Answer from the drawing. Dimensions are ordinates in mm from the lowest x, y and z of the part. A direction names the side the tool comes from. Give positions to 0.01 mm unless a question says otherwise; leave off trailing zeros. Loops run counter-clockwise (first coordinate to the right, second up) from the corner with the lowest first, then second, coordinate; pieces in that order, holes last.
Item 1: Section C-C, the plane z = 2 is taken. Give the vertices of the cut face in (x, y).
Item 2: Section D-D, the plane x = 58.5 is taken. Give the vertices of the cut face in (y, z), and give its area (3 significant figures).
Item 3: Section A-A, the plane y = 11.5 is taken. Give the vertices of the cut face in (x, z), and give its area (3 significant figures).
Item 4: Section B-B, the plane z = 9 is taken. Give the vertices of the cut face in (x, y).
Item 5: Consider line 1 along X through (y, z) = (28.5, 2.5); line 2 along Y through (x, z) = (72, 2.5); line 3 along X through (y, z) = (23.5, 7). Determine where each line is inside the solid, lowest interval first.
Item 6: The mould has two halves that part along X. Classify the marked faces 1, 2, 3 and 4: pulls with the +X half, pulls with the -X half, needs draft (parallel to the pull), parting line crosses it, or undercut.
Item 7: Each of these flat-tipped pins is pushed along its axis until it touches: pin 1 Ø4 at (x, y) = (72, 6.5) entering from +Z; pin 2 Ø6 at (y, z) = (25, 4.5) entering from +X; pin 3 Ø3 at (x, z) = (3.5, 5) entering from +Y (3 decimals); pin 4 Ø3 at (y, z) = (16.5, 5) entering from +X. Where does it stop, or does it pass through?
Item 8: A tool of negligible diameter and unlimited length cuts with its end or side. For the marked faces 5, 6, 7, 8 and 9, from which of +Z, -Z, +X, -X, +Y, -Y can it reach the whole face along a straight path? Write none if from no direction.
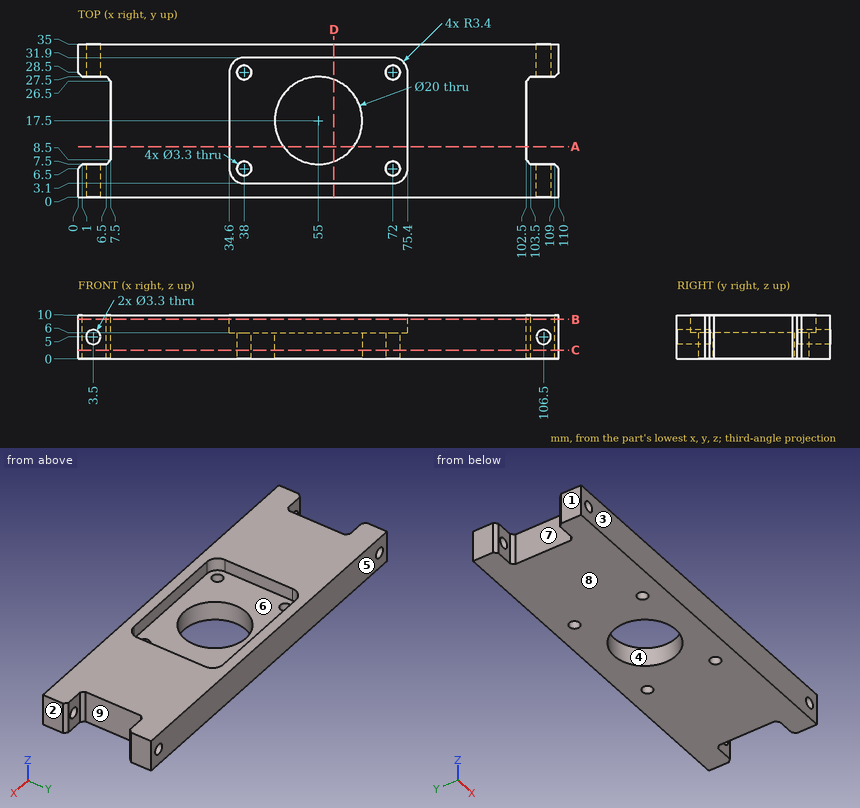
Worked answers:
1. outline: (0, 0) - (110, 0) - (110, 6.5) - (109, 7.5) - (103.5, 7.5) - (102.5, 8.5) - (102.5, 26.5) - (103.5, 27.5) - (109, 27.5) - (110, 28.5) - (110, 35) - (0, 35) - (0, 28.5) - (1, 27.5) - (6.5, 27.5) - (7.5, 26.5) - (7.5, 8.5) - (6.5, 7.5) - (1, 7.5) - (0, 6.5) - close; hole circle Ø3.3 at (38, 6.5); hole circle Ø3.3 at (38, 28.5); hole circle Ø20 at (55, 17.5); hole circle Ø3.3 at (72, 6.5); hole circle Ø3.3 at (72, 28.5)
2. outline: (0, 0) - (8.13, 0) - (8.13, 6) - (3.1, 6) - (3.1, 10) - (0, 10) - close; (26.87, 0) - (35, 0) - (35, 10) - (31.9, 10) - (31.9, 6) - (26.87, 6) - close
2. area: 122 mm2
3. outline: (7.5, 0) - (47, 0) - (47, 6) - (34.6, 6) - (34.6, 10) - (7.5, 10) - close; (63, 0) - (102.5, 0) - (102.5, 10) - (75.4, 10) - (75.4, 6) - (63, 6) - close
3. area: 691 mm2
4. outline: (0, 0) - (110, 0) - (110, 6.5) - (109, 7.5) - (103.5, 7.5) - (102.5, 8.5) - (102.5, 26.5) - (103.5, 27.5) - (109, 27.5) - (110, 28.5) - (110, 35) - (0, 35) - (0, 28.5) - (1, 27.5) - (6.5, 27.5) - (7.5, 26.5) - (7.5, 8.5) - (6.5, 7.5) - (1, 7.5) - (0, 6.5) - close; hole (34.6, 6.5) arc R3.4 ccw to (38, 3.1) - (72, 3.1) arc R3.4 ccw to (75.4, 6.5) - (75.4, 28.5) arc R3.4 ccw to (72, 31.9) - (38, 31.9) arc R3.4 ccw to (34.6, 28.5) - close
5. line 1: x = 0 to 36.35, 39.65 to 70.35, 73.65 to 110
5. line 2: y = 0 to 4.85, 8.15 to 26.85, 30.15 to 35
5. line 3: x = 7.5 to 34.6, 75.4 to 102.5
6. face 1: pulls with the -X half
6. face 2: pulls with the +X half
6. face 3: needs draft
6. face 4: undercut
7. pin 1: stops at z = 6
7. pin 2: stops at x = 109.5
7. pin 3: passes through
7. pin 4: stops at x = 102.5
8. face 5: +Z, -Z, +X, -X, +Y
8. face 6: +Z
8. face 7: +Z, -Z, -X
8. face 8: -Z, +X, -X, +Y, -Y
8. face 9: +Z, -Z, +X
